Input: part model. Units: mm. Frame: model coordinates. A direction names the side the tool comes from. Coordinates: 2 decimals unless noted, no trailing zeros. Loops run counter-clockwise (first coordinate to the right, second up) from the corner with the lowest first, then second, coordinate; pieces in that order, holes last. Notation, with made-up numbers: M -21.5,25 L 3.5,25 A14 ccw 3.5,32 Z; hole C 12.25,20.5 d5. An arc over 180 degrees is marked long. Use a Markdown table: item, result. Add a question column.
1. Pin query (flat end, axial travel): pin 1 (3 mm diameter, centred on x = 51.5, y = -9.5, fed in from +Z); pin 2 (4 mm diameter, centred on x = 79, z = 6.5, fed in from +Y); pin 3 (0.6 mm diameter, centred on x = 47.5, y = -1.5, fed in from +Z). Return the tip coordinate at first contact, or that it passes through.
2. Draft query along X for faces 1 (the flat face through (100, -6, 20)), 2 (the flat face through (50, -1, 19)), 3 (the flat face through (49, -12, 15)), 4 (the flat face through (0, -6, 20)). Return one class per face: +X half, -X half, draft (parallel to the pull), parting line (faces both ways), or undercut.
3. Line query: L1, parallel to X at y = -3.5, z = 36; L2, parallel to Z at x = 23.5, y = -3.25; L3, parallel to X at y = -1.25, z = 26.5. Output: solid intervals per line, ascending. Write a range as [from, to].
4. Section A-A on z = 33.5. Output: boundary loops of the cut face in (x, y).
5. Section D-D on z = 6.5. Output: boundary loops of the cut face in (x, y).
6. Section C-C on y = -9.5. Output: boundary loops of the cut face in (x, z), then the cut area to 3 significant figures.
7. Section B-B on x = 25. Output: boundary loops of the cut face in (y, z).
8. Set-up query: faces 5 (the flat face through (79, -6, 40)), 6 (the cylindrical face through (60.1, -7.07, 17.36)), 7 (the flat face through (41.9, -1, 31)). Return all of +Z, -Z, +X, -X, +Y, -Y with unobstructed straight access to the full face (end or side cutting, diameter ignored); none if empty.
```python
from build123d import *

# Parameters (mm, degrees)
F0_W     = 100
F0_H     = 12
F1_DEPTH = 40
F2_R     = 2.5
F3_DEPTH = 25
F5_DEPTH = 10
F7_DEPTH = 25


with BuildPart() as f1:
    # F0 (on Top) → F1 (new body)
    with BuildSketch(Plane.XY):
        with Locations((50, -6)):
            Rectangle(F0_W, F0_H)
    extrude(amount=F1_DEPTH)

    # F2 (on face) → F3 (cut)
    with BuildSketch(Plane.XZ.offset(12)):
        with Locations((79, 6.5)):
            Circle(F2_R)
        with Locations((23.5, 6.5)):
            Circle(F2_R)
    extrude(amount=-F3_DEPTH, mode=Mode.SUBTRACT)

    # F4 (on face) → F5 (cut)
    with BuildSketch(Plane.XZ.offset(12)):
        with BuildLine():
            Line((61, 40), (39, 40))
            Line((39, 40), (39, 19.5))
            ThreePointArc((39, 19.5), (39.87868, 17.37868), (42, 16.5))
            Line((42, 16.5), (58, 16.5))
            ThreePointArc((58, 16.5), (60.12132, 17.37868), (61, 19.5))
            Line((61, 19.5), (61, 40))
        make_face()
    extrude(amount=-F5_DEPTH, mode=Mode.SUBTRACT)

    # F6 (on face) → F7 (cut)
    with BuildSketch(Plane.XZ.offset(2)):
        with BuildLine():
            Line((58.1, 40), (41.9, 40))
            Line((41.9, 40), (41.9, 22))
            ThreePointArc((41.9, 22), (42.77868, 19.87868), (44.9, 19))
            Line((44.9, 19), (55.1, 19))
            ThreePointArc((55.1, 19), (57.22132, 19.87868), (58.1, 22))
            Line((58.1, 22), (58.1, 40))
        make_face()
    extrude(amount=-F7_DEPTH, mode=Mode.SUBTRACT)


solid = f1.part
```
Answers below:
| question | item | result |
|---|---|---|
| 1 | pin 1 | stops at z = 16.5 |
| 1 | pin 2 | passes through |
| 1 | pin 3 | stops at z = 19 |
| 2 | face 1 | +X half |
| 2 | face 2 | undercut |
| 2 | face 3 | draft |
| 2 | face 4 | -X half |
| 3 | L1 | x = [0, 39], [61, 100] |
| 3 | L2 | z = [0, 4], [9, 40] |
| 3 | L3 | x = [0, 41.9], [58.1, 100] |
| 4 | outline | M 0,-12 L 39,-12 L 39,-2 L 41.9,-2 L 41.9,0 L 0,0 Z; M 58.1,-2 L 61,-2 L 61,-12 L 100,-12 L 100,0 L 58.1,0 Z |
| 5 | outline | M 0,-12 L 21,-12 L 21,0 L 0,0 Z; M 26,-12 L 76.5,-12 L 76.5,0 L 26,0 Z; M 81.5,-12 L 100,-12 L 100,0 L 81.5,0 Z |
| 6 | outline | M 0,0 L 100,0 L 100,40 L 61,40 L 61,19.5 A3 cw 58,16.5 L 42,16.5 A3 cw 39,19.5 L 39,40 L 0,40 Z; hole C 23.5,6.5 d5; hole C 79,6.5 d5 |
| 6 | area | 3,450 mm² |
| 7 | outline | M -12,0 L 0,0 L 0,4.5 L -12,4.5 Z; M -12,8.5 L 0,8.5 L 0,40 L -12,40 Z |
| 8 | face 5 | +Z, +X, -X, +Y, -Y |
| 8 | face 6 | +Z, -Y |
| 8 | face 7 | +Z, +Y, -Y |
